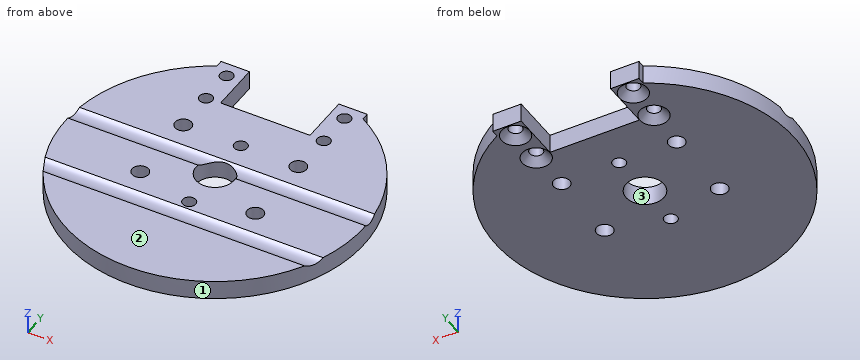
from build123d import *

# Parameters (mm, degrees)
SKETCH1_R               = 50
EXTRUDE_1_4_DEPTH       = 6.35
CUT_EXTRUDE1_DEPTH      = 6.35
SKETCH3_W               = 9.525
SKETCH3_H               = 16.75
BOSS_EXTRUDE2_DEPTH     = 6.35
SKETCH4_R               = 2.2
M4_THROUGH_DEPTH        = 6.35
SKETCH5_R               = 6.35
CUT_EXTRUDE2_DEPTH      = 6.35
SKETCH6_R               = 2.2
M4_THROUGH2_DEPTH       = 6.35
SKETCH7_R               = 2.75
M5_THROUGH_DEPTH        = 6.35
CHAMFER1_SIZE           = 2.5
CUT_EXTRUDE4_DEPTH      = 71.995228713
CUT_EXTRUDE4_DEPTH_BACK = 71.995228713
SKETCH8_R               = 5


with BuildPart() as part:
    # Sketch1 → 1/4 (new body)
    with BuildSketch(Plane.XY):
        Circle(SKETCH1_R)
    extrude(amount=EXTRUDE_1_4_DEPTH)

    # Sketch2 → Cut-Extrude1 (cut)
    with BuildSketch(Plane.XY.offset(6.35)):
        Polygon((-15, 46), (-15, 29.25), (15, 29.25), (15, 46), (28.100203936, 46), (28.100203936, 76.142415264), (-30.736146894, 76.142415264), (-30.736146894, 46), align=None)
    extrude(amount=-CUT_EXTRUDE1_DEPTH, mode=Mode.SUBTRACT)

    # Sketch3 → Boss-Extrude2 (add)
    with BuildSketch(Plane.XY.offset(6.35)):
        with Locations((-19.7625, 37.625)):
            Rectangle(SKETCH3_W, SKETCH3_H)
        with Locations((19.7625, 37.625)):
            Rectangle(SKETCH3_W, SKETCH3_H)
    extrude(amount=-BOSS_EXTRUDE2_DEPTH)

    # Sketch4 → M4_through (cut)
    with BuildSketch(Plane.XY.offset(6.35)):
        with Locations((-19.7625, 41)):
            Circle(SKETCH4_R)
        with Locations((-19.7625, 29)):
            Circle(SKETCH4_R)
        with Locations((19.7625, 29)):
            Circle(SKETCH4_R)
        with Locations((19.7625, 41)):
            Circle(SKETCH4_R)
    extrude(amount=-M4_THROUGH_DEPTH, mode=Mode.SUBTRACT)

    # Sketch5 → Cut-Extrude2 (cut)
    with BuildSketch(Plane.XY.offset(6.35)):
        Circle(SKETCH5_R)
    extrude(amount=-CUT_EXTRUDE2_DEPTH, mode=Mode.SUBTRACT)

    # Sketch6 → M4_through2 (cut)
    with BuildSketch(Plane.XY.offset(6.35)):
        with Locations((0, 15)):
            Circle(SKETCH6_R)
        with Locations((0, -15)):
            Circle(SKETCH6_R)
    extrude(amount=-M4_THROUGH2_DEPTH, mode=Mode.SUBTRACT)

    # Sketch7 → M5_through (cut)
    with BuildSketch(Plane.XY.offset(6.35)):
        with Locations((-19.3, 15)):
            Circle(SKETCH7_R)
        with Locations((-19.3, -10)):
            Circle(SKETCH7_R)
        with Locations((19.3, -10)):
            Circle(SKETCH7_R)
        with Locations((19.3, 15)):
            Circle(SKETCH7_R)
    extrude(amount=-M5_THROUGH_DEPTH, mode=Mode.SUBTRACT)

    # Chamfer1
    chamfer1_edges = [part.edges().sort_by_distance(p)[0] for p in [
        (17.5625, 41, 0),
        (17.5625, 29, 0),
        (-21.9625, 29, 0),
        (-21.9625, 41, 0),
    ]]
    chamfer(chamfer1_edges, length=CHAMFER1_SIZE)

    # Sketch8 → Cut-Extrude4 (cut, two sides: drawn at the far end of the back side and taken through both)
    with BuildSketch(Plane(origin=(0, 0, 0), x_dir=(0, 0, -1), z_dir=(1, 0, 0)).offset(-CUT_EXTRUDE4_DEPTH_BACK)):
        with Locations((-10.35, 4)):
            Circle(SKETCH8_R)
        with Locations((-10.35, -21)):
            Circle(SKETCH8_R)
    extrude(amount=CUT_EXTRUDE4_DEPTH + CUT_EXTRUDE4_DEPTH_BACK, mode=Mode.SUBTRACT)


solid = part.part
The model under review builds one solid part; all positions refer to its coordinate system, in mm. Face numbers are marked on the shaded views. Give positions to 0.01 mm unless a question says otherwise; leave off trailing zeros. Order: outer loops, then holes, each group sorted by start corner. A loop starts at its lowest first (then second) coordinate and runs counter-clockwise, first axis right, second up. Notation, with made-up numbers: M 65.5,-11.75 L 116.5,-11.75 A24 cw 116.5,11.25 Z; hole C 65.5,25 d3. An arc over 180 degrees is marked long. One line per question, with ' | ' between items. Start each with the question number.
1) Wall thickness on L1, parallel to X at y = 40, z = 1; L2, parallel to Y at x = 19.3, z = 4.75; L3, parallel to Y at x = 7, z = 1.25: over which ranges is each line inside the solid? List them lowest first. Write a range as from..to.
2) Clearance check with flat-ended pins moving along their axes: P1, Ø3.5, axis at x = 0, y = 15, coming from the -Z side; P2, Ø3, axis at y = 19.5, z = 2, coming from the +X side; P3, Ø2.5, axis at y = 45, z = 3.5, coming from the +X side (3 decimals); P4, Ø1.2, axis at y = 45.5, z = 3, coming from the -X side (3 decimals). State where each tip first meets the part, or that it passes through.
3) Consider section B-B, the plane x = 0. Give the boundary of the cut face in (y, z).
4) Consider section A-A, the plane y = -10. Give the boundary of the cut face in (x, z), then the cut area to 3 significant figures.
5) Consider section D-D, the plane x = 39.5. Give the boundary of the cut face in (y, z).
6) Consider section C-C, the plane y = 15. Give the boundary of the cut face in (x, z).
7) Mouldability with a two-part tool opening along Y and no side actions: class the marked faces 1, 2 and 3 as pulls with the +Y half, pulls with the -Y half, needs draft (parallel to the pull), parting line crosses it, or undercut.
Found:
1) L1: x = -30..-23.32, -16.2..-15, 15..16.2, 23.32..30 | L2: y = -46.12..-12.75, -7.25..12.25, 17.75..26.85, 31.15..38.85, 43.15..46 | L3: y = -49.51..29.25
2) P1: passes through | P2: stops at x = 46.65 | P3: stops at x = 24.525 | P4: stops at x = -24.525
3) outline: M -50,0 L -17.2,0 L -17.2,6.35 L -18,6.35 A5 cw -24,6.35 L -50,6.35 Z; M -12.8,0 L -6.35,0 L -6.35,6.35 L -12.8,6.35 Z; M 6.35,0 L 12.8,0 L 12.8,6.35 L 7,6.35 A5 cw 6.35,5.94 Z; M 17.2,0 L 29.25,0 L 29.25,6.35 L 17.2,6.35 Z
4) outline: M -48.99,0 L -22.05,0 L -22.05,6.35 L -48.99,6.35 Z; M -16.55,0 L 16.55,0 L 16.55,6.35 L -16.55,6.35 Z; M 22.05,0 L 48.99,0 L 48.99,6.35 L 22.05,6.35 Z | area: 552 mm²
5) outline: M -30.66,0 L 30.66,0 L 30.66,6.35 L 7,6.35 A5 cw 1,6.35 L -18,6.35 A5 cw -24,6.35 L -30.66,6.35 Z
6) outline: M -47.7,0 L -22.05,0 L -22.05,6.35 L -47.7,6.35 Z; M -16.55,0 L -2.2,0 L -2.2,6.35 L -16.55,6.35 Z; M 2.2,0 L 16.55,0 L 16.55,6.35 L 2.2,6.35 Z; M 22.05,0 L 47.7,0 L 47.7,6.35 L 22.05,6.35 Z
7) face 1: parting line crosses it | face 2: needs draft | face 3: undercut
